from build123d import *

# Parameters (mm, degrees)
SKETCH_1_R           = 12
SKETCH_1_R_2         = 6
EXTRUDE_1_DEPTH      = 30
SKETCH_2_R           = 6
SKETCH_2_R_2         = 2.25
EXTRUDE_2_DEPTH      = 10
EXTRUDE_START        = -36
SKETCH_23_W          = 30
SKETCH_23_H          = 50
SKETCH_23_R          = 2.25
EXTRUDE_10_DEPTH     = 36
SKETCH_24_W          = 30
SKETCH_24_H          = 8
CUT_EXTRUDE_16_DEPTH = 66.76473219
SKETCH_25_R          = 12
CUT_EXTRUDE_17_DEPTH = 47.324939288
SKETCH_26_R          = 2
CUT_EXTRUDE_18_DEPTH = 10


with BuildPart() as part:
    # Sketch 1 → Extrude 1 (new body)
    with BuildSketch(Plane(origin=(0, 0, 0), x_dir=(1, 0, 0), z_dir=(0, 1, 0))):
        with Locations(Location((0, 0, 0), (0, 0, 270))):
            Circle(SKETCH_1_R)
        with Locations(Location((0, 0, 0), (0, 0, 270))):
            Circle(SKETCH_1_R_2, mode=Mode.SUBTRACT)
    extrude(amount=EXTRUDE_1_DEPTH)

    # Sketch 2 → Extrude 2 (add)
    with BuildSketch(Plane(origin=(0, 30, 0), x_dir=(1, 0, 0), z_dir=(0, 1, 0))):
        with BuildLine():
            Line((-15, 13.228756555), (-15, -13.228756555))
            ThreePointArc((-15, -13.228756555), (0, -20), (15, -13.228756555))
            Line((15, -13.228756555), (15, 13.228756555))
            ThreePointArc((15, 13.228756555), (0, 20), (-15, 13.228756555))
        make_face()
        with Locations(Location((0, 0, 0), (0, 0, 270))):
            Circle(SKETCH_2_R, mode=Mode.SUBTRACT)
        with Locations(Location((0, 16, 0), (0, 0, 270))):
            Circle(SKETCH_2_R_2, mode=Mode.SUBTRACT)
        with Locations(Location((11.313708499, 11.313708499, 0), (0, 0, 270))):
            Circle(SKETCH_2_R_2, mode=Mode.SUBTRACT)
        with Locations(Location((11.313708499, -11.313708499, 0), (0, 0, 270))):
            Circle(SKETCH_2_R_2, mode=Mode.SUBTRACT)
        with Locations(Location((0, -16, 0), (0, 0, 270))):
            Circle(SKETCH_2_R_2, mode=Mode.SUBTRACT)
        with Locations(Location((-11.313708499, -11.313708499, 0), (0, 0, 270))):
            Circle(SKETCH_2_R_2, mode=Mode.SUBTRACT)
        with Locations(Location((-11.313708499, 11.313708499, 0), (0, 0, 270))):
            Circle(SKETCH_2_R_2, mode=Mode.SUBTRACT)
    extrude(amount=EXTRUDE_2_DEPTH)

    # Sketch 23 → Extrude 10 (add)
    with BuildSketch(Plane(origin=(0, 40, 0), x_dir=(1, 0, 0), z_dir=(0, 1, 0)).offset(EXTRUDE_START)):
        Rectangle(SKETCH_23_W, SKETCH_23_H)
        with Locations(Location((-11.313708499, -11.313708499, 0), (0, 0, 270))):
            Circle(SKETCH_23_R, mode=Mode.SUBTRACT)
        with Locations(Location((0, -16, 0), (0, 0, 270))):
            Circle(SKETCH_23_R, mode=Mode.SUBTRACT)
        with Locations(Location((11.313708499, -11.313708499, 0), (0, 0, 270))):
            Circle(SKETCH_23_R, mode=Mode.SUBTRACT)
        with Locations(Location((11.313708499, 11.313708499, 0), (0, 0, 270))):
            Circle(SKETCH_23_R, mode=Mode.SUBTRACT)
        with Locations(Location((0, 16, 0), (0, 0, 270))):
            Circle(SKETCH_23_R, mode=Mode.SUBTRACT)
        with Locations(Location((-11.313708499, 11.313708499, 0), (0, 0, 270))):
            Circle(SKETCH_23_R, mode=Mode.SUBTRACT)
    extrude(amount=EXTRUDE_10_DEPTH)

    # Sketch 24 → Cut-Extrude 16 (cut, through all)
    with BuildSketch(Plane.XY.offset(25)):
        Rectangle(SKETCH_24_W, SKETCH_24_H)
    extrude(amount=-CUT_EXTRUDE_16_DEPTH, mode=Mode.SUBTRACT)

    # Sketch 25 → Cut-Extrude 17 (cut, through all)
    with BuildSketch(Plane(origin=(0, 40, 0), x_dir=(1, 0, 0), z_dir=(0, 1, 0))):
        with Locations(Location((0, 0, 0), (0, 0, 270))):
            Circle(SKETCH_25_R)
    extrude(amount=-CUT_EXTRUDE_17_DEPTH, mode=Mode.SUBTRACT)

    # Sketch 26 → Cut-Extrude 18 (cut)
    with BuildSketch(Plane(origin=(15, 0, 0), x_dir=(0, 0, -1), z_dir=(1, 0, 0))):
        with Locations((17.5, 34)):
            Circle(SKETCH_26_R)
        with Locations((-17.5, 34)):
            Circle(SKETCH_26_R)
        with Locations((-17.5, 10)):
            Circle(SKETCH_26_R)
        with Locations((17.5, 10)):
            Circle(SKETCH_26_R)
    extrude(amount=-CUT_EXTRUDE_18_DEPTH, mode=Mode.SUBTRACT)


solid = part.part
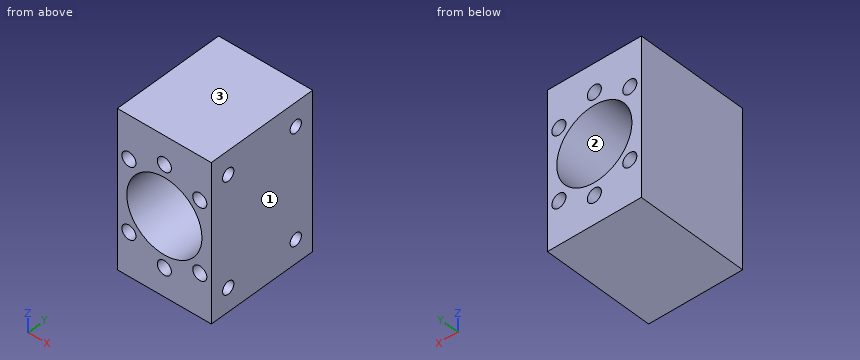
Model file for the job. Use its own axes, mm. Face numbers are marked on the shaded views. Give positions to 0.01 mm unless a question says otherwise; leave off trailing zeros. Order: outer loops, then holes, each group sorted by start corner. A loop starts at its lowest first (then second) coordinate and runs counter-clockwise, first axis right, second up. Notation, with made-up numbers: M -28.5,84.25 L -7.5,84.25 A18 cw -7.5,89.25 Z; hole C -34,0.25 d1. An arc over 180 degrees is marked long. Put each result on its own line as item: value. Start each with the question number.
(1) Pull direction X, two halves, no side cores. Call the marked faces 1, 2 and 3: released by +X, released by -X, zero draft, split by the parting line, or undercut.
(2) Band-saw the part on A-A on x = 10.25. Give the cut face in (y, z), then the cut area to 3 significant figures.
(3) Band-saw the part on B-B on z = 0. Give the cut face in (x, y).
(4) Band-saw the part on C-C on y = 33. Give the cut face in (x, z).
(5) Drill centre lines: L1, parallel to Y at x = 12, z = -17.5; L2, parallel to Z at x = -10, y = 19.5; L3, parallel to Z at x = 9.25, y = 15.5. Where is each one in solid material? Low to high. Write a range as [from, to].
(6) Band-saw the part on D-D on z = -6.5. Give the cut face in (x, y).
Results below:
1. face 1: released by +X
1. face 2: undercut
1. face 3: zero draft
2. outline: M 4,-25 L 40,-25 L 40,-13.3 L 4,-13.3 Z; M 4,-9.33 L 40,-9.33 L 40,-6.24 L 4,-6.24 Z; M 4,6.24 L 40,6.24 L 40,9.33 L 4,9.33 Z; M 4,13.3 L 40,13.3 L 40,25 L 4,25 Z; hole C 10,-17.5 d4; hole C 10,17.5 d4; hole C 34,-17.5 d4; hole C 34,17.5 d4
2. area: 1,010 mm2
3. outline: M -15,4 L -12,4 L -12,40 L -15,40 Z; M 12,4 L 15,4 L 15,40 L 12,40 Z
4. outline: M -15,-25 L 15,-25 L 15,-19.23 L 5,-19.23 L 5,-15.77 L 15,-15.77 L 15,15.77 L 5,15.77 L 5,19.23 L 15,19.23 L 15,25 L -15,25 Z; hole C -11.31,-11.31 d4.5; hole C -11.31,11.31 d4.5; hole C 0,0 d24; hole C 0,-16 d4.5; hole C 0,16 d4.5; hole C 11.31,-11.31 d4.5; hole C 11.31,11.31 d4.5
5. L1: y = [4, 8], [12, 32], [36, 40]
5. L2: z = [-25, -13.14], [-9.49, -6.63], [6.63, 9.49], [13.14, 25]
5. L3: z = [-25, -12.21], [-10.42, -7.64], [7.64, 10.42], [12.21, 25]
6. outline: M -15,4 L -10.09,4 L -10.09,40 L -15,40 Z; M 10.09,4 L 15,4 L 15,40 L 10.09,40 Z
